from build123d import *

# Parameters (mm, degrees)
F1_DEPTH = 5.334
F2_R     = 1.143
F3_DEPTH = 25.4


with BuildPart() as f1:
    # F0 (on Front) → F1 (new body)
    with BuildSketch(Plane.XZ):
        with BuildLine():
            Line((433.180757, 21.996105), (-81.169243, 21.996105))
            ThreePointArc((-81.169243, 21.996105), (-85.659371, 20.136233), (-87.519243, 15.646105))
            Line((-87.519243, 15.646105), (-87.519243, -44.043895))
            ThreePointArc((-87.519243, -44.043895), (-85.659371, -48.534023), (-81.169243, -50.393895))
            Line((-81.169243, -50.393895), (312.530757, -50.393895))
            ThreePointArc((312.530757, -50.393895), (317.020885, -52.253767), (318.880757, -56.743895))
            Line((318.880757, -56.743895), (318.880757, -84.580526))
            ThreePointArc((318.880757, -84.580526), (320.740629, -89.070654), (325.230757, -90.930526))
            Line((325.230757, -90.930526), (331.580757, -90.930526))
            ThreePointArc((331.580757, -90.930526), (336.070885, -89.070654), (337.930757, -84.580526))
            Line((337.930757, -84.580526), (337.930757, -56.743895))
            ThreePointArc((337.930757, -56.743895), (339.790629, -52.253767), (344.280757, -50.393895))
            Line((344.280757, -50.393895), (433.180757, -50.393895))
            ThreePointArc((433.180757, -50.393895), (437.670885, -48.534023), (439.530757, -44.043895))
            Line((439.530757, -44.043895), (439.530757, -18.643895))
            Line((439.530757, -18.643895), (414.130757, -18.643895))
            Line((414.130757, -18.643895), (414.130757, -12.801895))
            Line((414.130757, -12.801895), (439.530757, -12.801895))
            Line((439.530757, -12.801895), (439.530757, 15.646105))
            ThreePointArc((439.530757, 15.646105), (437.670885, 20.136233), (433.180757, 21.996105))
        make_face()
    extrude(amount=F1_DEPTH)

    # F2 (on face) → F3 (cut)
    with BuildSketch(Plane.XZ.offset(5.334)):
        with Locations((-68.469243, -14.833895)):
            Circle(F2_R)
    extrude(amount=-F3_DEPTH, mode=Mode.SUBTRACT)


solid = f1.part
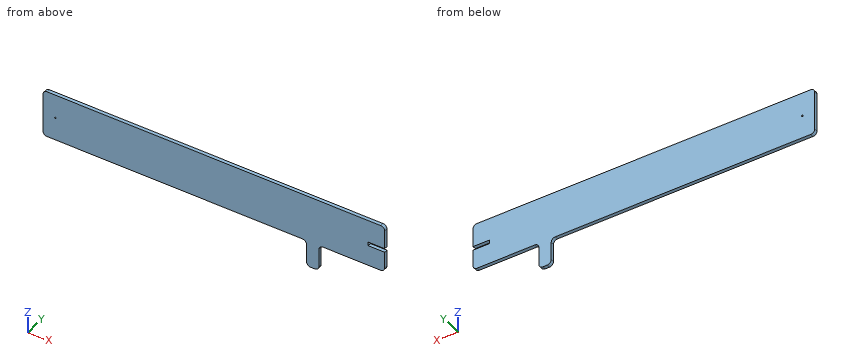
Verification items for the finished model (mm, model axes). Give positions to 0.01 mm unless a question says otherwise; leave off trailing zeros. Loops run counter-clockwise (first coordinate to the right, second up) from the corner with the lowest first, then second, coordinate; pieces in that order, holes last.
1. Cross-section at B-B on z = -78. Record the cut outline in (x, y), and give its area (3 significant figures).
Derived:
outline: (318.88, -5.33) - (337.93, -5.33) - (337.93, 0) - (318.88, 0) - close
area: 102 mm2
2. Cross-section at C-C on x = 284. Record the cut outline in (y, z), and give its area (3 significant figures).
Derived:
outline: (-5.33, -50.39) - (0, -50.39) - (0, 22) - (-5.33, 22) - close
area: 386 mm2
3. Material ranges on probe 1 along Z at (x, y) = (359, -0.5); probe 2 along X at (y, z) = (-1.65, -65); probe 3 along X at (y, z) = (-0.3, -48), recorded low to high.
Derived:
probe 1: z = -50.39 to 22
probe 2: x = 318.88 to 337.93
probe 3: x = -86.14 to 438.15
4. Cross-section at A-A on y = -2.4. Record the cut outline in (x, z), and give its area (3 significant figures).
Derived:
outline: (-87.52, -44.04) arc R6.35 ccw to (-81.17, -50.39) - (312.53, -50.39) arc R6.35 cw to (318.88, -56.74) - (318.88, -84.58) arc R6.35 ccw to (325.23, -90.93) - (331.58, -90.93) arc R6.35 ccw to (337.93, -84.58) - (337.93, -56.74) arc R6.35 cw to (344.28, -50.39) - (433.18, -50.39) arc R6.35 ccw to (439.53, -44.04) - (439.53, -18.64) - (414.13, -18.64) - (414.13, -12.8) - (439.53, -12.8) - (439.53, 15.65) arc R6.35 ccw to (433.18, 22) - (-81.17, 22) arc R6.35 ccw to (-87.52, 15.65) - close; hole circle Ø2.29 at (-68.47, -14.83)
area: 38,700 mm2
5. Go/stop test with flat-tipped pins: P1, Ø2.5, axis at x = 377.5, y = -2, coming from the -Z side; P2, Ø2, axis at y = -2.5, z = -76, coming from the +X side; P3, Ø1.6, axis at y = -2.5, z = -75, coming from the -X side. Record where each tip stops, or that it passes through.
Derived:
P1: stops at z = -50.39
P2: stops at x = 337.93
P3: stops at x = 318.88
